from build123d import *

# Parameters (mm, degrees)
EXTRUDE_1_DEPTH          = 110
SKETCH_3_W               = 5
SKETCH_3_H               = 20
EXTRUDE_2_DEPTH          = 110
CUT_EXTRUDE_1_REACH      = 232.418
SKETCH_2_R               = 2.25
SKETCH_5_W               = 5
SKETCH_5_H               = 50.5
CUT_EXTRUDE_2_DEPTH      = 234.512847612
SKETCH_6_W               = 29.75
SKETCH_6_H               = 157
CUT_EXTRUDE_3_DEPTH      = 10
SKETCH_7_W               = 3
SKETCH_7_H               = 145
EXTRUDE_3_DEPTH          = 6
FILLET_1_R               = 1
CHAMFER_1_SIZE           = 8
CHAMFER_2_SIZE           = 4
SKETCH_8_R               = 1.7
CUT_EXTRUDE_4_DEPTH      = 232.154169333
CUT_EXTRUDE_5_DEPTH      = 13
CUT_EXTRUDE_5_DEPTH_BACK = 13
CHAMFER_3_SIZE           = 12
CHAMFER_3_SIZE_2         = 6.92820323
CHAMFER_4_SIZE           = 5.196152423
CHAMFER_4_SIZE_2         = 3


with BuildPart() as part:
    # 草图1 → 凸台-拉伸1 (new body)
    with BuildSketch(Plane.XY):
        Polygon((0, 0), (20.5, 0), (20.5, -196), (14.5, -196), (14.5, -200), (23.5, -200), (23.5, 4), (-3, 4), (-3, -43), (0, -43), align=None)
    extrude(amount=EXTRUDE_1_DEPTH)

    # 草图3 → 凸台-拉伸2 (add)
    with BuildSketch(Plane(origin=(0, 0, 0), x_dir=(-1, 0, 0), z_dir=(0, 0, -1))):
        with Locations((-26, -33)):
            Rectangle(SKETCH_3_W, SKETCH_3_H)
        with Locations((5.5, -33)):
            Rectangle(SKETCH_3_W, SKETCH_3_H)
    extrude(amount=-EXTRUDE_2_DEPTH)

    # 草图2 → 切除-拉伸1 (cut, up to next)
    with BuildSketch(Plane(origin=(23.5, 0, 0), x_dir=(0, 0, -1), z_dir=(1, 0, 0)), mode=Mode.PRIVATE) as cut_extrude_1_sk1:
        with Locations(Location((-55, -38.5, 0), (0, 0, 90))):
            Circle(SKETCH_2_R)
    cut_extrude_1_tool1 = extrude(cut_extrude_1_sk1.sketch, amount=-CUT_EXTRUDE_1_REACH, mode=Mode.PRIVATE) & part.part
    # 草图2 → 切除-拉伸1 (cut, up to next)
    with BuildSketch(Plane(origin=(23.5, 0, 0), x_dir=(0, 0, -1), z_dir=(1, 0, 0)), mode=Mode.PRIVATE) as cut_extrude_1_sk2:
        with Locations(Location((-55, -183.5, 0), (0, 0, 90))):
            Circle(SKETCH_2_R)
    cut_extrude_1_tool2 = extrude(cut_extrude_1_sk2.sketch, amount=-CUT_EXTRUDE_1_REACH, mode=Mode.PRIVATE) & part.part
    add(cut_extrude_1_tool1.solids().sort_by_distance((23.5, -38.5, 55))[0], mode=Mode.SUBTRACT)
    add(cut_extrude_1_tool2.solids().sort_by_distance((23.5, -183.5, 55))[0], mode=Mode.SUBTRACT)

    # 草图5 → 切除-拉伸2 (cut, through all)
    with BuildSketch(Plane(origin=(0, 4, 0), x_dir=(1, 0, 0), z_dir=(0, 1, 0))):
        with Locations((-5.5, -55)):
            Rectangle(SKETCH_5_W, SKETCH_5_H)
        with Locations((26, -55)):
            Rectangle(SKETCH_5_W, SKETCH_5_H)
    extrude(amount=-CUT_EXTRUDE_2_DEPTH, mode=Mode.SUBTRACT)

    # 草图6 → 切除-拉伸3 (cut)
    with BuildSketch(Plane(origin=(23.5, 0, 0), x_dir=(0, 0, -1), z_dir=(1, 0, 0))):
        with Locations((-95.125, -121.5)):
            Rectangle(SKETCH_6_W, SKETCH_6_H)
        with Locations((-14.875, -121.5)):
            Rectangle(SKETCH_6_W, SKETCH_6_H)
    extrude(amount=-CUT_EXTRUDE_3_DEPTH, mode=Mode.SUBTRACT)

    # 草图7 → 凸台-拉伸3 (add)
    with BuildSketch(Plane.ZY.offset(-20.5)):
        with Locations((31.25, -123.5)):
            Rectangle(SKETCH_7_W, SKETCH_7_H)
        with Locations((78.75, -123.5)):
            Rectangle(SKETCH_7_W, SKETCH_7_H)
    extrude(amount=EXTRUDE_3_DEPTH)

    # 圆角1
    fillet_1_edges = [part.edges().sort_by_distance(p)[0] for p in [
        (23.5, -200, 55),
        (14.5, -200, 55),
        (-3, 4, 55),
        (23.5, 4, 55),
        (14.5, -196, 55),
        (20.5, -196, 55),
        (-3, -43, 55),
    ]]
    fillet(fillet_1_edges, radius=FILLET_1_R)

    # 倒角1
    chamfer_1_edges = [part.edges().sort_by_distance(p)[0] for p in [
        (22, -43, 80.25),
        (22, -43, 29.75),
    ]]
    chamfer(chamfer_1_edges, length=CHAMFER_1_SIZE)

    # 倒角2
    # the kernel refuses this chamfer: 4 mm, written as the material it adds along each edge
    with BuildSketch(Plane(origin=(-3, -23, 29.75), x_dir=(0.027495876610586726, 0, 0.9996219169112968), z_dir=(0, -1, 0))) as chamfer_2_piece_1:
        Polygon((CHAMFER_2_SIZE * 0.999621916911, CHAMFER_2_SIZE * 0.0274958766106), (-CHAMFER_2_SIZE * 0.0274958766106, CHAMFER_2_SIZE * 0.999621916911), (0, 0), align=None)
    extrude(amount=19)
    with BuildSketch(Plane(origin=(-3, -23, 80.25), x_dir=(0.027495876610584242, 0, -0.9996219169112968), z_dir=(0, -1, 0))) as chamfer_2_piece_2:
        Polygon((CHAMFER_2_SIZE * 0.999621916911, -CHAMFER_2_SIZE * 0.0274958766106), (-CHAMFER_2_SIZE * 0.0274958766106, -CHAMFER_2_SIZE * 0.999621916911), (0, 0), align=None)
    extrude(amount=19)
    with BuildSketch(Plane(origin=(-2, -42, 29.75), x_dir=(-0.9999802608561371, 0.0062831439655610674, 0), z_dir=(-0.0062831439655610674, -0.9999802608561371, 0))) as chamfer_2_piece_3_section:
        Polygon((-1 - CHAMFER_2_SIZE, 0), (-1, -CHAMFER_2_SIZE), (-1, 0), align=None)
    chamfer_2_piece_3 = revolve(axis=Axis((-2, -42, 29.75), (0, 0, -1)), revolution_arc=359.64, mode=Mode.PRIVATE)
    chamfer_2_piece_3 = split(chamfer_2_piece_3, bisect_by=Plane(origin=(0, -42.77460492, 31.688294831), z_dir=(-1, 0, 0)), keep=Keep.TOP, mode=Mode.PRIVATE)
    chamfer_2_piece_3 = split(chamfer_2_piece_3, bisect_by=Plane(origin=(-2.77460492, -43, 31.688294831), z_dir=(0, 1, 0)), keep=Keep.TOP, mode=Mode.PRIVATE)
    add(chamfer_2_piece_3)
    with BuildSketch(Plane(origin=(-2, -42, 80.25), x_dir=(-0.9999802608561371, 0.0062831439655610674, 0), z_dir=(-0.0062831439655610674, -0.9999802608561371, 0))) as chamfer_2_piece_4_section:
        Polygon((-1, CHAMFER_2_SIZE), (-1 - CHAMFER_2_SIZE, 0), (-1, 0), align=None)
    chamfer_2_piece_4 = revolve(axis=Axis((-2, -42, 80.25), (0, 0, -1)), revolution_arc=359.64, mode=Mode.PRIVATE)
    chamfer_2_piece_4 = split(chamfer_2_piece_4, bisect_by=Plane(origin=(0, -42.77460492, 78.31170517), z_dir=(-1, 0, 0)), keep=Keep.TOP, mode=Mode.PRIVATE)
    chamfer_2_piece_4 = split(chamfer_2_piece_4, bisect_by=Plane(origin=(-2.77460492, -43, 78.31170517), z_dir=(0, 1, 0)), keep=Keep.TOP, mode=Mode.PRIVATE)
    add(chamfer_2_piece_4)
    with BuildSketch(Plane(origin=(23.5, -23, 80.25), x_dir=(-0.027495876610602904, 0, -0.9996219169112963), z_dir=(0, -1, 0))) as chamfer_2_piece_5:
        Polygon((CHAMFER_2_SIZE * 0.999621916911, CHAMFER_2_SIZE * 0.0274958766106), (-CHAMFER_2_SIZE * 0.0274958766106, CHAMFER_2_SIZE * 0.999621916911), (0, 0), align=None)
    extrude(amount=20)
    with BuildSketch(Plane(origin=(23.5, -23, 29.75), x_dir=(-0.02749587661060549, 0, 0.9996219169112961), z_dir=(0, -1, 0))) as chamfer_2_piece_6:
        Polygon((CHAMFER_2_SIZE * 0.999621916911, -CHAMFER_2_SIZE * 0.0274958766106), (-CHAMFER_2_SIZE * 0.0274958766106, -CHAMFER_2_SIZE * 0.999621916911), (0, 0), align=None)
    extrude(amount=20)

    # 草图8 → 切除-拉伸4 (cut, through all)
    with BuildSketch(Plane.ZY.offset(8)):
        with Locations(Location((15, -33.335006201, 0), (0, 0, 270))):
            Circle(SKETCH_8_R)
        with Locations(Location((95, -33.335006201, 0), (0, 0, 270))):
            Circle(SKETCH_8_R)
    extrude(amount=-CUT_EXTRUDE_4_DEPTH, mode=Mode.SUBTRACT)

    # 草图9 → 切除-拉伸5 (cut, two sides: drawn at the far end of the back side and taken through both)
    with BuildSketch(Plane(origin=(10.25, 0, 0), x_dir=(0, 0, -1), z_dir=(1, 0, 0)).offset(-CUT_EXTRUDE_5_DEPTH_BACK)):
        Polygon((-93.354551733, -30.485006201), (-96.645448267, -30.485006201), (-98.290896534, -33.335006201), (-96.645448267, -36.185006201), (-93.354551733, -36.185006201), (-91.709103466, -33.335006201), align=None)
        Polygon((-13.354551733, -30.485006201), (-16.645448267, -30.485006201), (-18.290896534, -33.335006201), (-16.645448267, -36.185006201), (-13.354551733, -36.185006201), (-11.709103466, -33.335006201), align=None)
    extrude(amount=CUT_EXTRUDE_5_DEPTH + CUT_EXTRUDE_5_DEPTH_BACK, mode=Mode.SUBTRACT)

    # 倒角3
    # the kernel refuses this chamfer: 12, 6.92820323 mm, written as the material it takes off along each edge
    with BuildSketch(Plane(origin=(14.5, -51, 111.295029056), x_dir=(-0.019326765612700716, -0.9998132206222078, -4.736066806866801e-15), z_dir=(0, 0, -1))) as chamfer_3_piece_1_section:
        Polygon((CHAMFER_3_SIZE * 0.999813220622, -CHAMFER_3_SIZE * 0.0193267656127), (-CHAMFER_3_SIZE_2 * 0.0193267656135, -CHAMFER_3_SIZE_2 * 0.999813220662), (0, 0), align=None)
    chamfer_3_piece_1 = extrude(amount=65.090058112, mode=Mode.PRIVATE)
    chamfer_3_piece_1 = split(chamfer_3_piece_1, bisect_by=Plane(origin=(20.5, -55.138426071, 78.75), z_dir=(-1, 0, 0)), keep=Keep.TOP, mode=Mode.PRIVATE)
    add(chamfer_3_piece_1, mode=Mode.SUBTRACT)
    with BuildSketch(Plane(origin=(14.5, -51, 63.795029056), x_dir=(0.9983227437537925, 0.0578938624026711, 0), z_dir=(0, 0, -1))) as chamfer_3_piece_2_section:
        Polygon((CHAMFER_3_SIZE_2 * 0.998322743793, CHAMFER_3_SIZE_2 * 0.057893862405), (-CHAMFER_3_SIZE * 0.0578938624027, CHAMFER_3_SIZE * 0.998322743754), (0, 0), align=None)
    chamfer_3_piece_2 = extrude(amount=65.090058112, mode=Mode.PRIVATE)
    chamfer_3_piece_2 = split(chamfer_3_piece_2, bisect_by=Plane(origin=(20.5, -55.138426071, 31.25), z_dir=(-1, 0, 0)), keep=Keep.TOP, mode=Mode.PRIVATE)
    add(chamfer_3_piece_2, mode=Mode.SUBTRACT)

    # 倒角4
    # the kernel refuses this chamfer: 5.196152423, 3 mm, written as the material it takes off along each edge
    with BuildSketch(Plane(origin=(0, -43, 123.442891912), x_dir=(0.01932676561270063, 0.9998132206222079, 0), z_dir=(0, 0, -1))) as chamfer_4_piece_1:
        Polygon((CHAMFER_4_SIZE * 0.999813220566, -CHAMFER_4_SIZE * 0.0193267656116), (-CHAMFER_4_SIZE_2 * 0.0193267656127, -CHAMFER_4_SIZE_2 * 0.999813220622), (0, 0), align=None)
    extrude(amount=136.885783824, mode=Mode.SUBTRACT)


solid = part.part
Verification items for the finished model (mm, model axes). A direction names the side the tool comes from. Give positions to 0.01 mm unless a question says otherwise; leave off trailing zeros. Loops run counter-clockwise (first coordinate to the right, second up) from the corner with the lowest first, then second, coordinate; pieces in that order, holes last. Notation, with made-up numbers: (1.25, 68) - (23.25, 68) arc R30 ccw to (23.25, 104) - close; hole circle Ø6 at (5.5, -33). An arc over 180 degrees is marked (long way). Write item = value, one per line. Start each with the question number.
Q1. Tool access check on faces 1 (the face through (22.02, -38.79, 57.23)), 2 (the face through (14.5, -131, 32)), 3 (the face through (-3, -14, 56)), 4 (the face through (20.5, -74, 54)). Record the directions out of +Z, -Z, +X, -X, +Y, -Y that give a thin tool (end or side, any length) a straight path to the whole face; none if there is none.
Q2. Cross-section at D-D, the plane z = 39.5. Enter the section's corners in (x, y), and give its area (3 significant figures).
Q3. Mould release check, pull along X, two halves, no side actions. Record for faces 5 (the face through (25.47, -32.86, 78.22)), 6 (the face through (22.02, -46.94, 25.69)), 7 (the face through (0, -19, 56)): released by +X, released by -X, zero draft, split by the parting line, or undercut.
Q4. Cross-section at A-A, the plane z = 55. Enter the section's corners in (x, y).
Q5. Depth check by flat-ended pin: P1, Ø1.5, axis at x = -5, z = 95.5, coming from the -Y side; P2, Ø2, axis at y = -94.5, z = 67, coming from the +X side; P3, Ø1, axis at y = -171.5, z = 31, coming from the -X side; P4, Ø2, axis at y = -33.34, z = 95, coming from the +X side. Enter the tip coordinate at first touch or a pass-through.
Q6. Cross-section at C-C, the plane y = -183.5. Enter the section's corners in (x, z), and give its area (3 significant figures).
Q7. Cross-section at B-B, the plane y = -124.5. Enter the section's corners in (x, z).
Q8. Thickness scan on line 1 (Y direction, x = 24.95, z = 95) (3 decimals); line 2 (Z direction, x = 22, y = -38.5); line 3 (Z direction, x = 18.5, y = -176.5). Record the ranges inside material, lowest first.
Answer key:
q1.face_1 = +X
q1.face_2 = +Z, -Z, -X, -Y
q1.face_3 = -X, +Y
q1.face_4 = none
q2.outline = (-3, -42) arc R1 ccw to (-2.78, -42.62) - (0, -37.8) - (0, 0) - (20.5, 0) - (20.5, -195) arc R1 cw to (19.5, -196) - (15.5, -196) arc R1 ccw to (14.5, -197) - (14.5, -199) arc R1 ccw to (15.5, -200) - (22.5, -200) arc R1 ccw to (23.5, -199) - (23.5, 3) arc R1 ccw to (22.5, 4) - (-2, 4) arc R1 ccw to (-3, 3) - close
q2.area = 850 mm^2
q3.face_5 = released by +X
q3.face_6 = zero draft
q3.face_7 = undercut
q4.outline = (-3, -42) arc R1 ccw to (-2.78, -42.62) - (0, -37.8) - (0, 0) - (20.5, 0) - (20.5, -36.25) - (23.5, -36.25) - (23.5, 3) arc R1 ccw to (22.5, 4) - (-2, 4) arc R1 ccw to (-3, 3) - close; (14.5, -199) arc R1 ccw to (15.5, -200) - (22.5, -200) arc R1 ccw to (23.5, -199) - (23.5, -185.75) - (20.5, -185.75) - (20.5, -195) arc R1 cw to (19.5, -196) - (15.5, -196) arc R1 ccw to (14.5, -197) - close; (20.5, -181.25) - (23.5, -181.25) - (23.5, -40.75) - (20.5, -40.75) - close
q5.P1 = -43
q5.P2 = 23.5
q5.P3 = 14.5
q5.P4 = through
q6.outline = (14.5, 29.75) - (23.5, 29.75) - (23.5, 52.75) - (20.5, 52.75) - (20.5, 32.75) - (14.5, 32.75) - close; (14.5, 77.25) - (20.5, 77.25) - (20.5, 57.25) - (23.5, 57.25) - (23.5, 80.25) - (14.5, 80.25) - close
q6.area = 174 mm^2
q7.outline = (14.5, 29.75) - (23.5, 29.75) - (23.5, 80.25) - (14.5, 80.25) - (14.5, 77.25) - (20.5, 77.25) - (20.5, 32.75) - (14.5, 32.75) - close
q8.line_1 = -43 to -35.035, -31.635 to -23
q8.line_2 = 0 to 52.75, 57.25 to 110
q8.line_3 = 29.75 to 32.75, 77.25 to 80.25
